```python
from build123d import *

# Parameters (mm, degrees)
SKETCH1_R           = 4.7625
BOSS_EXTRUDE1_DEPTH = 3
BOSS_EXTRUDE2_DEPTH = 3
FILLET1_R           = 1
SKETCH4_R           = 20
CUT_EXTRUDE1_DEPTH  = 10
FILLET2_R           = 2.5


with BuildPart() as part:
    # Sketch1 → Boss-Extrude1 (new body)
    with BuildSketch(Plane(origin=(0, 0, 0), x_dir=(1, 0, 0), z_dir=(0, 1, 0))):
        with BuildLine():
            Line((-31.819805153, 31.819805153), (-7.071067812, 7.071067812))
            ThreePointArc((-7.071067812, 7.071067812), (0, 10), (7.071067812, 7.071067812))
            Line((7.071067812, 7.071067812), (31.819805153, 31.819805153))
            ThreePointArc((31.819805153, 31.819805153), (0, -45), (-31.819805153, 31.819805153))
        make_face()
        Circle(SKETCH1_R, mode=Mode.SUBTRACT)
    extrude(amount=BOSS_EXTRUDE1_DEPTH)

    # Sketch3 → Boss-Extrude2 (add)
    with BuildSketch(Plane(origin=(0, 3, 0), x_dir=(1, 0, 0), z_dir=(0, 1, 0))):
        Polygon((-31.819805153, 31.819805153), (-27.577164466, 36.062445841), (-27.577164466, 27.577164466), align=None)
        Polygon((27.577164466, 27.577164466), (31.819805153, 31.819805153), (27.577164466, 36.062445841), align=None)
    extrude(amount=-BOSS_EXTRUDE2_DEPTH)

    # Fillet1
    fillet1_edges = [part.edges().sort_by_distance(p)[0] for p in [
        (-27.577164466, 1.5, -27.577164466),
        (27.577164466, 1.5, -27.577164466),
        (7.071067812, 1.5, -7.071067812),
        (-7.071067812, 1.5, -7.071067812),
    ]]
    fillet(fillet1_edges, radius=FILLET1_R)

    # Sketch4 → Cut-Extrude1 (cut)
    with BuildSketch(Plane(origin=(0, 3, 0), x_dir=(1, 0, 0), z_dir=(0, 1, 0))):
        with Locations((-47.631397208, -27.5)):
            Circle(SKETCH4_R)
        with Locations((47.631397208, -27.5)):
            Circle(SKETCH4_R)
        with Locations((0, -55)):
            Circle(SKETCH4_R)
    extrude(amount=-CUT_EXTRUDE1_DEPTH, mode=Mode.SUBTRACT)

    # Fillet2
    fillet2_edges = [part.edges().sort_by_distance(p)[0] for p in [
        (15.427784317, 1.5, 42.272727273),
        (-15.427784317, 1.5, 42.272727273),
        (44.323147864, 1.5, 7.775510494),
        (28.895363547, 1.5, 34.497216779),
        (-28.895363547, 1.5, 34.497216779),
        (-44.323147864, 1.5, 7.775510494),
    ]]
    fillet(fillet2_edges, radius=FILLET2_R)


solid = part.part
```
Verification items for the finished model (mm, model axes). A direction names the side the tool comes from. Give positions to 0.01 mm unless a question says otherwise; leave off trailing zeros. Loops run counter-clockwise (first coordinate to the right, second up) from the corner with the lowest first, then second, coordinate; pieces in that order, holes last.
1. Mould release check, pull along Z, two halves, no side actions. Record for faces 3 (the flat face through (29.73, 1.52, -33.91)), 4 (the flat face through (27.577, 2, -32)), 5 (the cylindrical face through (-3.78, 1.48, 2.9)): released by +Z, released by -Z, zero draft, split by the parting line, or undercut.
2. Thickness scan on line 1 (X direction, y = 1.85, z = 0); line 2 (X direction, y = 0.5, z = -16); line 3 (Z direction, x = -8, y = 2). Record the ranges inside material, lowest first.
3. Section check C-C, the plane z = 26.5. Enter the section's corners in (x, y).
4. Set-up check for faces 1 (the cylindrical face through (0, 2, 35)), 2 (the flat face through (-27.577, 2, -32)): record each of +Z, -Z, +X, -X, +Y, -Y from which the full face is reachable in a straight line by a thin tool's end or side.
5. Section check B-B, the plane z = 0. Enter the section's corners in (x, y), then the cut area to 3 significant figures.
6. Section check D-D, the plane x = 22.5. Enter the section's corners in (y, z), then the cut area to 3 significant figures.
7. Go/stop test with flat-tipped pins: pin 1 Ø1.5 at (y, z) = (2.5, 4.5) entering from -X; pin 2 Ø1.5 at (y, z) = (1.5, 22.5) entering from +X; pin 3 Ø8.5 at (x, z) = (0, 0) entering from +Y; pin 4 Ø1 at (y, z) = (1, 21) entering from -X. Record where each tip stops, or that it passes through.
8. Section check A-A, the plane x = 0. Enter the section's corners in (y, z).
Geometry says:
1. face 3: released by -Z
1. face 4: zero draft
1. face 5: undercut
2. line 1: x = -45 to -4.76, 4.76 to 45
2. line 2: x = -42.06 to -16, 16 to 42.06
2. line 3: z = -8 to 36.67
3. outline: (-27.66, 0) - (27.66, 0) - (27.66, 3) - (-27.66, 3) - close
4. face 1: +Z, +Y, -Y
4. face 2: -Z, +Y, -Y
5. outline: (-45, 0) - (-4.76, 0) - (-4.76, 3) - (-45, 3) - close; (4.76, 0) - (45, 0) - (45, 3) - (4.76, 3) - close
5. area: 241 mm2
6. outline: (0, -22.5) - (3, -22.5) - (3, 38.97) - (0, 38.97) - close
6. area: 184 mm2
7. pin 1: stops at x = -44.84
7. pin 2: stops at x = 28.48
7. pin 3: passes through
7. pin 4: stops at x = -28.9
8. outline: (0, -10) - (3, -10) - (3, -4.76) - (0, -4.76) - close; (0, 4.76) - (3, 4.76) - (3, 35) - (0, 35) - close
